```python
from build123d import *

# Parameters (mm, degrees)
SKETCH2_W           = 210
SKETCH2_H           = 150
BOSS_EXTRUDE3_DEPTH = 275
SKETCH5_W           = 204
SKETCH5_H           = 144
CUT_EXTRUDE1_DEPTH  = 272
SKETCH6_W           = 210
SKETCH6_H           = 275
CUT_EXTRUDE2_DEPTH  = 3
BOSS_EXTRUDE4_DEPTH = 3
BOSS_EXTRUDE6_DEPTH = 210
CUT_EXTRUDE3_DEPTH  = 210
SKETCH12_R          = 3
SKETCH12_W          = 7
SKETCH12_H          = 12
CUT_EXTRUDE4_DEPTH  = 26


with BuildPart() as part:
    # Sketch2 → Boss-Extrude3 (new body)
    with BuildSketch(Plane(origin=(0, 0, 0), x_dir=(1, 0, 0), z_dir=(0, 1, 0))):
        with Locations((49.81119073, 12.425134533)):
            Rectangle(SKETCH2_W, SKETCH2_H)
    extrude(amount=BOSS_EXTRUDE3_DEPTH)

    # Sketch5 → Cut-Extrude1 (cut)
    with BuildSketch(Plane(origin=(0, 275, 0), x_dir=(1, 0, 0), z_dir=(0, 1, 0))):
        with Locations((49.81119073, 12.425134533)):
            Rectangle(SKETCH5_W, SKETCH5_H)
    extrude(amount=-CUT_EXTRUDE1_DEPTH, mode=Mode.SUBTRACT)

    # Sketch6 → Cut-Extrude2 (cut)
    with BuildSketch(Plane.XY.offset(62.574865467)):
        with Locations((49.81119073, 137.5)):
            Rectangle(SKETCH6_W, SKETCH6_H)
    extrude(amount=-CUT_EXTRUDE2_DEPTH, mode=Mode.SUBTRACT)

    # Sketch8 → Boss-Extrude4 (add)
    with BuildSketch(Plane(origin=(0, 275, 0), x_dir=(1, 0, 0), z_dir=(0, 1, 0))):
        Polygon((154.81119073, -62.574865467), (123.063521966, -62.574865467), (123.063521966, 36.23081547), (-48.18880927, 36.23081547), (-48.18880927, -62.574865467), (-55.18880927, -62.574865467), (-55.18880927, 87.425134533), (154.81119073, 87.425134533), align=None)
    extrude(amount=BOSS_EXTRUDE4_DEPTH)

    # Sketch10 → Boss-Extrude6 (add)
    with BuildSketch(Plane(origin=(154.81119073, 0, 0), x_dir=(0, 0, -1), z_dir=(1, 0, 0))):
        Polygon((87.425134533, 278), (232.314008477, 316.822856765), (232.314008477, 286.822856765), (87.425134533, 218), align=None)
    extrude(amount=-BOSS_EXTRUDE6_DEPTH)

    # Sketch11 → Cut-Extrude3 (cut)
    with BuildSketch(Plane(origin=(0, 237.521247493, 63.643626451), x_dir=(-1, 0, 0), z_dir=(0, 0.9659258262890681, 0.25881904510252135))):
        Polygon((-19.81119073, -306.397889851), (55.18880927, -156.397889851), (55.18880927, -306.397889851), align=None)
        Polygon((-79.81119073, -306.397889851), (-154.81119073, -156.397889851), (-154.81119073, -306.397889851), align=None)
    extrude(amount=-CUT_EXTRUDE3_DEPTH, mode=Mode.SUBTRACT)

    # Sketch12 → Cut-Extrude4 (cut)
    with BuildSketch(Plane(origin=(154.81119073, 0, 0), x_dir=(0, 0, -1), z_dir=(1, 0, 0))):
        with Locations((-39.574865467, 30)):
            Circle(SKETCH12_R)
        with Locations((-39.074865467, 56)):
            Rectangle(SKETCH12_W, SKETCH12_H)
    extrude(amount=-CUT_EXTRUDE4_DEPTH, mode=Mode.SUBTRACT)


solid = part.part
```
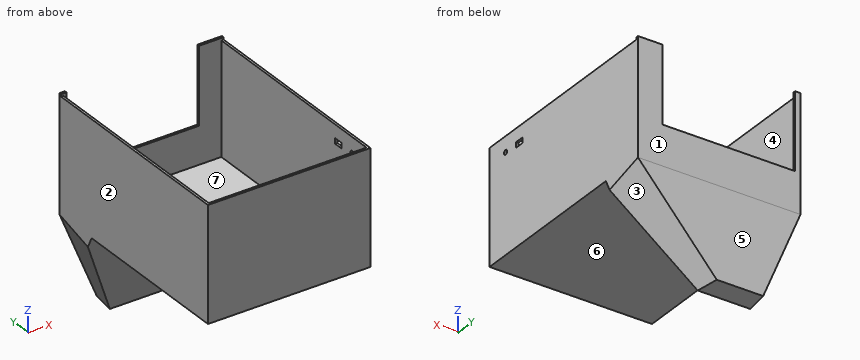
Input: part model. Units: mm. Frame: model coordinates. Face numbers are marked on the shaded views. A direction names the side the tool comes from. Give positions to 0.01 mm unless a question says otherwise; leave off trailing zeros. Order: outer loops, then holes, each group sorted by start corner. A loop starts at its lowest first (then second) coordinate and runs counter-clockwise, first axis right, second up. Notation, with made-up numbers: (51.5, 4) - (59.5, 4) arc R19 ccw to (59.5, 37) - close; hole circle Ø6 at (20.25, -9). An arc over 180 degrees is marked (long way). Put each result on its own line as item: value.
Item 1: Draft query along X for the marked faces 1, 2, 3 and 4. Return one class per face: +X half, -X half, draft (parallel to the pull), parting line (faces both ways), or undercut.
Found:
face 1: draft
face 2: -X half
face 3: +X half
face 4: undercut
Item 2: Contact query for flat-ended pins moving along their axis: pin 1 (2 mm diameter, centred on x = -13.5, y = 204, fed in from +Z); pin 2 (1 mm diameter, centred on x = 12, y = 121, fed in from -Z); pin 3 (5 mm diameter, centred on x = 46, y = 226, fed in from -Z). Output: stop coordinate, or through.
Found:
pin 1: stops at z = -84.43
pin 2: stops at z = -87.43
pin 3: stops at z = -109.53
Item 3: Ray query, L1, parallel to X at y = 109.5, z = 12.5; L2, parallel to Y at x = -8, z = -59.5; L3, parallel to Z at x = -4.5, y = 83.5. Return the intervals inside material, ascending. Write a range as from..to.
Found:
L1: x = -55.19..-52.19, 151.81..154.81
L2: y = 0..3, 275..278
L3: z = -87.43..-84.43
Item 4: Section query C-C, the plane z = -143.5. Return loops of the section in (x, y).
Found:
outline: (-32.42, 244.64) - (132.05, 244.64) - (125.78, 293.03) - (-26.16, 293.03) - close
Item 5: Section query D-D, the plane z = -195. Return loops of the section in (x, y), then the cut area to 3 significant figures.
Found:
outline: (-4.39, 269.1) - (104.01, 269.1) - (99.13, 306.82) - (0.5, 306.82) - close
area: 3,910 mm^2
Item 6: Access query for the marked faces 5, 6 and 7. Directions: +Z, -Z, +X, -X, +Y, -Y. A direction counts if a zero-diameter tool reaches every point of the face in a straight line with its end or side. Return the directions, or none.
Found:
face 5: +Z, +X, -X, +Y
face 6: -Z, +X, -X, -Y
face 7: +Z
Item 7: Section query A-A, the plane x = 74.5. Return loops of the section in (y, z).
Found:
outline: (0, -87.43) - (218, -87.43) - (286.82, -232.31) - (316.82, -232.31) - (278, -87.43) - (278, -36.23) - (275, -36.23) - (275, -84.43) - (3, -84.43) - (3, 59.57) - (0, 59.57) - close
Item 8: Section query B-B, the plane x = -7. Return loops of the section in (y, z), then the cut area to 3 significant figures.
Found:
outline: (0, -87.43) - (218, -87.43) - (266.82, -190.2) - (302.94, -180.52) - (278, -87.43) - (278, -36.23) - (275, -36.23) - (275, -84.43) - (3, -84.43) - (3, 59.57) - (0, 59.57) - close
area: 6,300 mm^2
